```python
from build123d import *

# Parameters (mm, degrees)
F0_W      = 330.2
F0_H      = 254
F1_DEPTH  = 254
F2_T      = -7.62
F3_R      = 25.4
F4_DEPTH  = 25.4
F6_D      = 38.1
F6_DEPTH  = 76.2
F7_R      = 31.75
F8_DEPTH  = 25.4
F9_R      = 25.4
F10_DEPTH = 76.2


with BuildPart() as f1:
    # F0 (on Top) → F1 (new body)
    with BuildSketch(Plane.XY):
        Rectangle(F0_W, F0_H)
    extrude(amount=F1_DEPTH)

    # F2
    f2_openings = [f1.faces().sort_by_distance(p)[0] for p in [
        (0, 0, 254),
    ]]
    offset(amount=F2_T, openings=f2_openings)

    # F3 (on face) → F4 (join)
    with BuildSketch(Plane.YZ.offset(165.1)):
        with Locations((0, 31.760685)):
            Circle(F3_R)
    extrude(amount=F4_DEPTH)

    # F6
    with Locations(Plane.YZ.offset(190.5)):
        with Locations((0, 31.760685)):
            Hole(F6_D / 2, depth=F6_DEPTH)

    # F7 (on face) → F8 (join)
    with BuildSketch(Plane.XZ.offset(127)):
        with Locations((-107.95, 38.1)):
            Circle(F7_R)
    extrude(amount=F8_DEPTH)

    # F9 (on face) → F10 (cut)
    with BuildSketch(Plane.XZ.offset(152.4)):
        with Locations((-107.95, 38.1)):
            Circle(F9_R)
    extrude(amount=-F10_DEPTH, mode=Mode.SUBTRACT)


solid = f1.part
```
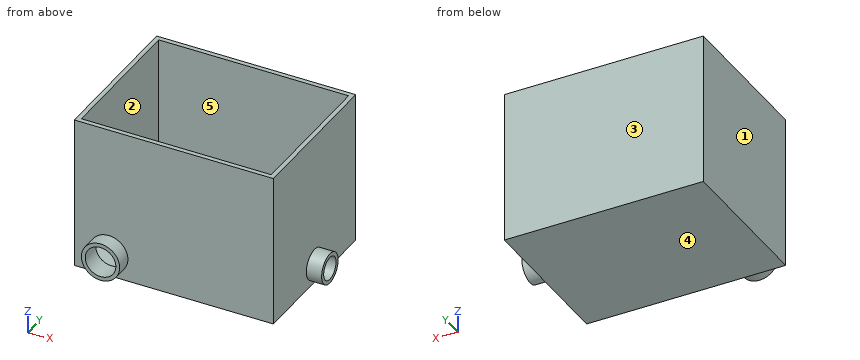
CAD build for the part. Positions are in the model's coordinates, mm. Face numbers are marked on the shaded views. A direction names the side the tool comes from. Round coordinates to 2 decimals unless told otherwise and drop trailing zeros. Write each loop counter-clockwise with the first axis right and the second up, starting at its lowest first coordinate (ties: lowest second). Pieces come first, ordered by that corner, then holes.
Item 1: Band-saw the part on A-A on y = 0. Write the cut outline in (x, z).
Filled in:
outline: (-165.1, 0) - (165.1, 0) - (165.1, 6.36) - (190.5, 6.36) - (190.5, 12.71) - (157.48, 12.71) - (157.48, 7.62) - (-157.48, 7.62) - (-157.48, 254) - (-165.1, 254) - close; (157.48, 50.81) - (190.5, 50.81) - (190.5, 57.16) - (165.1, 57.16) - (165.1, 254) - (157.48, 254) - close
Item 2: Tool access for the marked faces 4 and 5: list every direction of +Z, -Z, +X, -X, +Y, -Y with a clear straight run to the whole face (end or side of a thin tool).
Filled in:
face 4: -Z, +X, -X, +Y, -Y
face 5: +Z
Item 3: Drill centre lines: L1, parallel to Z at x = 165.5, y = 0; L2, parallel to X at y = 55.5, z = 19.5; L3, parallel to Y at x = -148.5, z = 11. Where is each one in solid material? Low to high.
Filled in:
L1: z = 6.36 to 12.71, 50.81 to 57.16
L2: x = -165.1 to -157.48, 157.48 to 165.1
L3: y = -127 to -119.38, 119.38 to 127
Item 4: Band-saw the part on D-D on x = 135.5. Write the cut outline in (y, z).
Filled in:
outline: (-127, 0) - (127, 0) - (127, 254) - (119.38, 254) - (119.38, 7.62) - (-119.38, 7.62) - (-119.38, 254) - (-127, 254) - close
Item 5: Band-saw the part on B-B on x = -107.95. Write the cut outline in (y, z), then the cut area to 3 significant figures.
Filled in:
outline: (-152.4, 6.35) - (-127, 6.35) - (-127, 0) - (127, 0) - (127, 254) - (119.38, 254) - (119.38, 7.62) - (-119.38, 7.62) - (-119.38, 12.7) - (-152.4, 12.7) - close; (-152.4, 63.5) - (-119.38, 63.5) - (-119.38, 254) - (-127, 254) - (-127, 69.85) - (-152.4, 69.85) - close
area: 5,630 mm2
Item 6: Drop flat-ended pins along their axis: pin 1 Ø10 at (x, z) = (-93, 175.5) entering from -Y; pin 2 Ø6 at (y, z) = (-97, 191) entering from +X; pin 3 Ø12 at (x, y) = (-40.5, 1.5) entering from +Z; pin 4 Ø5 at (x, y) = (85.5, -30.5) entering from -Z. Give the stop position or say it passes through.
Filled in:
pin 1: stops at y = -127
pin 2: stops at x = 165.1
pin 3: stops at z = 7.62
pin 4: stops at z = 0
Item 7: Band-saw the part on C-C on z = 174. Write the cut outline in (x, y), then the cut area to 3 significant figures.
Filled in:
outline: (-165.1, -127) - (165.1, -127) - (165.1, 127) - (-165.1, 127) - close; hole (-157.48, -119.38) - (157.48, -119.38) - (157.48, 119.38) - (-157.48, 119.38) - close
area: 8,670 mm2
Item 8: Mould opens along Y. For the marked faces 1, 2 and 3 say: released by +Y, released by -Y, zero draft, split by the parting line, or undercut.
Filled in:
face 1: zero draft
face 2: undercut
face 3: released by +Y
